from build123d import *

# Parameters (mm, degrees)
PAD_DEPTH           = 40
POCKET_DEPTH        = 105.001
SKETCH002_W         = 3.5
SKETCH002_H         = 24
POCKET001_DEPTH     = 35
LINEARPATTERN_COUNT = 12
LINEARPATTERN_PITCH = 8.181818
FILLET_R            = 2
CHAMFER_SIZE        = 2


with BuildPart() as part:
    # Sketch → Pad (new body)
    with BuildSketch(Plane.XY):
        with BuildLine():
            Line((-50, 22.5), (50, 22.5))
            ThreePointArc((52.5, 20), (51.767767, 21.767767), (50, 22.5))
            Line((52.5, 20), (52.5, -20))
            ThreePointArc((50, -22.5), (51.767767, -21.767767), (52.5, -20))
            Line((50, -22.5), (-50, -22.5))
            ThreePointArc((-52.5, -20), (-51.767767, -21.767767), (-50, -22.5))
            Line((-52.5, -20), (-52.5, 20))
            ThreePointArc((-50, 22.5), (-51.767767, 21.767767), (-52.5, 20))
        make_face()
    extrude(amount=PAD_DEPTH)

    # Sketch001 (on Face5 of Pad) → Pocket (cut, through all)
    with BuildSketch(Plane.YZ.offset(52.5)):
        with BuildLine():
            ThreePointArc((-34.433893, 0), (-12.512323, 19.11251), (0, 45.366749))
            Line((0, 45.366749), (-64.611679, 45.366749))
            Line((-64.611679, 45.366749), (-64.611679, 0))
            Line((-64.611679, 0), (-34.433893, 0))
        make_face()
    extrude(amount=-POCKET_DEPTH, mode=Mode.SUBTRACT)

    # Sketch002 (on Face4 of Pocket) → Pocket001 (cut)
    with BuildSketch(Plane.XY.offset(40)):
        with Locations((-43.75, -6)):
            Rectangle(SKETCH002_W, SKETCH002_H)
    pocket001 = extrude(amount=-POCKET001_DEPTH, mode=Mode.SUBTRACT)

    # LinearPattern: Pocket001 ×12
    with Locations(*[(i * LINEARPATTERN_PITCH, 0, 0) for i in range(1, LINEARPATTERN_COUNT)]):
        add(pocket001, mode=Mode.SUBTRACT)

    # Fillet
    fillet_edges = [part.edges().sort_by_distance(p)[0] for p in [
        (0, 22.5, 40),
    ]]
    fillet(fillet_edges, radius=FILLET_R)

    # Chamfer
    chamfer_edges = [part.edges().sort_by_distance(p)[0] for p in [
        (-50, 22.5, 19),
        (0, 22.5, 38),
        (0, 22.5, 0),
        (50, 22.5, 19),
        (-52.5, 0, 0),
        (-51.767767, 21.767767, 0),
        (51.767767, 21.767767, 0),
        (52.5, 0, 0),
        (51.767767, -21.767767, 0),
        (0, -22.5, 0),
        (-51.767767, -21.767767, 0),
    ]]
    chamfer(chamfer_edges, length=CHAMFER_SIZE)


solid = part.part
Read the model definition and answer for the solid it produces. Units are mm, in the model's axes. A direction names the side the tool comes from. Round coordinates to 2 decimals unless told otherwise and drop trailing zeros. Order: outer loops, then holes, each group sorted by start corner. A loop starts at its lowest first (then second) coordinate and runs counter-clockwise, first axis right, second up.
1) Flat-ended cylindrical pins translate along their axes: pin 1 (1.5 mm diameter, centred on x = -41.5, z = 13, fed in from -Y); pin 2 (1 mm diameter, centred on x = -6, z = 29, fed in from -Y); pin 3 (1.8 mm diameter, centred on x = -27, y = -11, fed in from +Z). Find the tip coordinate at first contact, or state that the pin passes through.
2) For faces 5 (the face through (-42, -4, 19)), 6 (the face through (51.062, -21.039, 0.986)), determine the directions among +Z, -Z, +X, -X, +Y, -Y from which every point of the face is accessible in a straight line to the end or side of a thin tool.
3) The mould has two halves that part along Y. Classify faces 1 (the face through (-36, -18, 9)), 2 (the face through (-27, 6, 23)), 3 (the face through (51.748, -21.787, 5.326)), 4 (the face through (-52.5, 4, 20)): released by +Y, released by -Y, zero draft, split by the parting line, or undercut.
4) The part is cut by section A-A on x = 37.5. Write down the section's boundary in (y, z) (3 decimals).
5) Straight lines are drawn through the part: L1, parallel to Y at x = -43, z = 22; L2, parallel to Z at x = 31, y = -10.5; L3, parallel to Y at x = -34, z = 7.5. For each, find the intervals that lie inside material, in ascending order.
6) The part is cut by section B-B on z = 9.5. Give the number of separate pieces and of enclosed holes in the cut face, plus the area to 3 significant figures.
Resolved:
1. pin 1: stops at y = -18.44
1. pin 2: stops at y = -6.48
1. pin 3: stops at z = 5
2. face 5: +Z
2. face 6: -Z, +X, -Y
3. face 1: undercut
3. face 2: undercut
3. face 3: released by -Y
3. face 4: zero draft
4. outline: (-22.5, 2) - (-20.5, 0) - (20.5, 0) - (22.5, 2) - (22.5, 38) arc R2 ccw to (20.5, 40) - (6, 40) - (6, 5) - (-18, 5) - (-18, 12.705) arc R71.605 cw to (-22.5, 8.425) - close
5. L1: y = 6 to 22.5
5. L2: z = 0 to 5
5. L3: y = -22.5 to -18, 6 to 22.5
6. separate pieces: 1
6. enclosed holes: 12
6. area: 3,590 mm2
